Source: three-view drawing plus pictorial views. Frame: mm from the lowest corner of the part. Give positions to 0.01 mm unless a question says otherwise; leave off trailing zeros. Order: outer loops, then holes, each group sorted by start corner. A loop starts at its lowest first (then second) coordinate and runs counter-clockwise, first axis right, second up.
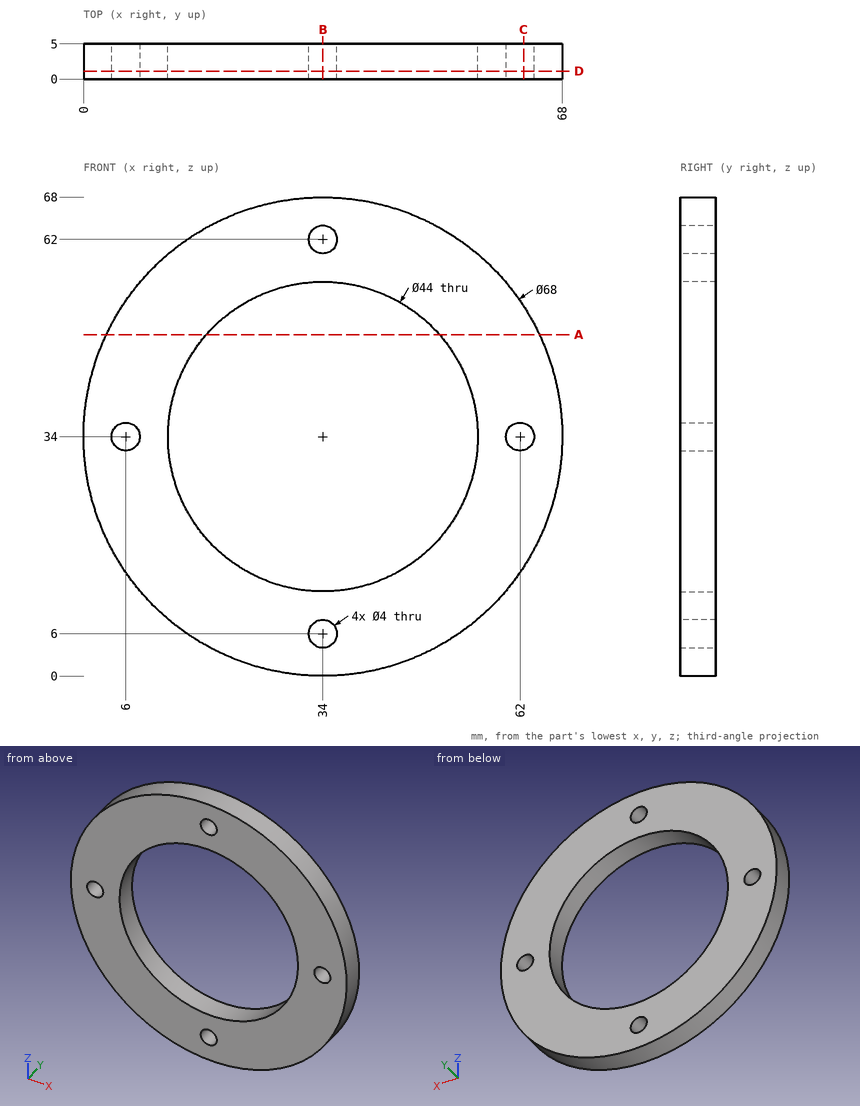
1) Ray query, L1, parallel to X at y = 2.5, z = 5.5; L2, parallel to X at y = 3, z = 46; L3, parallel to Z at x = 39, y = 3.85. Return the intervals inside material, ascending.
Checks:
L1: x = 15.46 to 32.06, 35.94 to 52.54
L2: x = 2.19 to 15.56, 52.44 to 65.81
L3: z = 0.37 to 12.58, 55.42 to 67.63
2) First-contact query: pin 1 Ø3.5 at (x, z) = (62, 34) entering from -Y; pin 2 Ø2 at (y, z) = (1.5, 19) entering from +X. Flat tips, straight axial feed; report the tip coordinate or a pass-through.
Checks:
pin 1: passes through
pin 2: stops at x = 64.98
3) Section query A-A on z = 48.5. Output: boundary loops of the cut face in (x, y).
Checks:
outline: (3.25, 0) - (17.45, 0) - (17.45, 5) - (3.25, 5) - close; (50.55, 0) - (64.75, 0) - (64.75, 5) - (50.55, 5) - close
4) Section query C-C on x = 62.5. Output: boundary loops of the cut face in (y, z), and give its area (3 significant figures).
Checks:
outline: (0, 15.46) - (5, 15.46) - (5, 32.06) - (0, 32.06) - close; (0, 35.94) - (5, 35.94) - (5, 52.54) - (0, 52.54) - close
area: 166 mm2
5) Section query D-D on y = 1.15. Output: boundary loops of the cut face in (x, z), and give its area (3 significant figures).
Checks:
outline: circle Ø68 at (34, 34); hole circle Ø4 at (6, 34); hole circle Ø44 at (34, 34); hole circle Ø4 at (34, 6); hole circle Ø4 at (34, 62); hole circle Ø4 at (62, 34)
area: 2,060 mm2
6) Section query B-B on x = 34. Output: boundary loops of the cut face in (y, z), and give its area (3 significant figures).
Checks:
outline: (0, 0) - (5, 0) - (5, 4) - (0, 4) - close; (0, 8) - (5, 8) - (5, 12) - (0, 12) - close; (0, 56) - (5, 56) - (5, 60) - (0, 60) - close; (0, 64) - (5, 64) - (5, 68) - (0, 68) - close
area: 80.0 mm2
